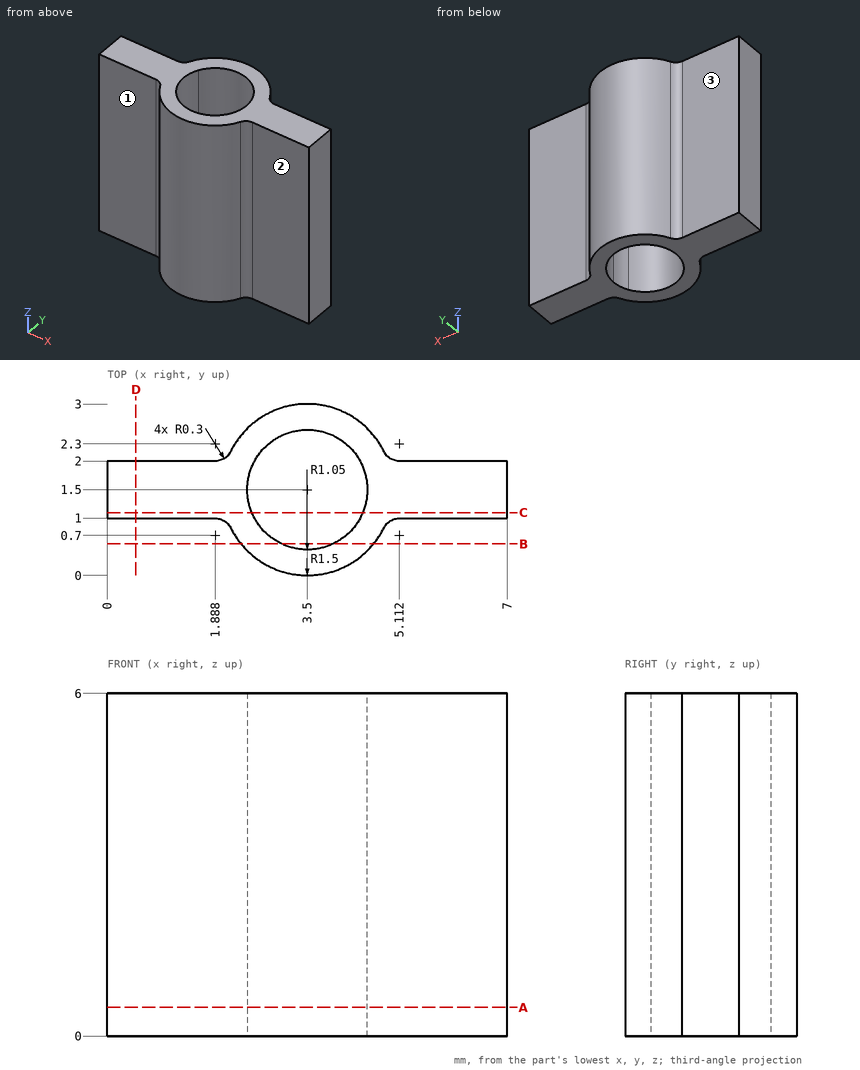
The figure shows three views and two pictorial views of one solid part (mm, origin at its lowest corner). Answer the questions. A direction names the side the tool comes from. Give positions to 0.01 mm unless a question says otherwise; leave off trailing zeros. Write each loop counter-clockwise with the first axis right and the second up, starting at its lowest first coordinate (ties: lowest second). Pieces come first, ordered by that corner, then holes. Notation, with made-up numbers: (13, 42) -> (17, 42) arc R19 cw to (17, 64) -> close; hole circle Ø5 at (46, -35.75). An arc over 180 degrees is marked (long way). Answer as a JSON object with one key per item and string values.
1) Section B-B on y = 0.55 is taken. Write down the section's boundary in (x, z).
Findings below:
{"outline": "(2.34, 0) -> (3.05, 0) -> (3.05, 6) -> (2.34, 6) -> close; (3.95, 0) -> (4.66, 0) -> (4.66, 6) -> (3.95, 6) -> close"}
2) Straight lines are drawn through the part: probe 1 along Y at (x, z) = (5.25, 0.6); probe 2 along Y at (x, z) = (4, 0.35) (1 decimal); probe 3 along X at (y, z) = (1.9, 2.35). For each, find the intervals that lie inside material, in ascending order. Write a range as from..to.
Findings below:
{"probe 1": "y = 1..2", "probe 2": "y = 0.1..0.6, 2.4..2.9", "probe 3": "x = 0..2.53, 4.47..7"}
3) Section A-A on z = 0.5 is taken. Write down the section's boundary in (x, y).
Findings below:
{"outline": "(0, 1) -> (1.89, 1) arc R0.3 cw to (2.16, 0.83) arc R1.5 ccw to (4.84, 0.83) arc R0.3 cw to (5.11, 1) -> (7, 1) -> (7, 2) -> (5.11, 2) arc R0.3 cw to (4.84, 2.17) arc R1.5 ccw to (2.16, 2.17) arc R0.3 cw to (1.89, 2) -> (0, 2) -> close; hole circle Ø2.1 at (3.5, 1.5)"}
4) Flat-ended cylindrical pins translate along their axes: pin 1 Ø0.9 at (x, z) = (1.5, 4.5) entering from +Y; pin 2 Ø1.5 at (x, y) = (5.5, 2.5) entering from -Z; pin 3 Ø0.9 at (x, z) = (6, 2) entering from -Y. Find the tip coordinate at first contact, or state that the pin passes through.
Findings below:
{"pin 1": "stops at y = 2.01", "pin 2": "stops at z = 0", "pin 3": "stops at y = 1"}
5) Section D-D on x = 0.5 is taken. Write down the section's boundary in (y, z).
Findings below:
{"outline": "(1, 0) -> (2, 0) -> (2, 6) -> (1, 6) -> close"}
6) Section C-C on y = 1.1 is taken. Write down the section's boundary in (x, z).
Findings below:
{"outline": "(0, 0) -> (2.53, 0) -> (2.53, 6) -> (0, 6) -> close; (4.47, 0) -> (7, 0) -> (7, 6) -> (4.47, 6) -> close"}
7) A tool of negligible diameter and unlimited length cuts with its end or side. For the marked faces 1, 2 and 3, from which of +Z, -Z, +X, -X, +Y, -Y can it reach the whole face along a straight path? Write none if from no direction.
Findings below:
{"face 1": "+Z, -Z, -X, -Y", "face 2": "+Z, -Z, +X, -Y", "face 3": "+Z, -Z, -X, +Y"}
